Could you check a few things on this model? Use its own coordinates, in mm. A direction names the side the tool comes from. Round coordinates to 2 decimals unless told otherwise and drop trailing zeros. Loops run counter-clockwise (first coordinate to the right, second up) from the corner with the lowest first, then second, coordinate; pieces in that order, holes last. Notation, with made-up numbers: (32.25, 87) -> (83.25, 87) arc R29 cw to (83.25, 110) -> close; hole circle Ø8 at (-21, 80.5). An arc over 180 degrees is marked (long way). One line per item, written item: value.
from build123d import *
from build123d.topology import SkipClean

# Parameters (mm, degrees)
SKETCH3_R           = 122.5
SKETCH3_R_2         = 118.5
EXTRUDE_THIN1_DEPTH = 192
SKETCH3_3_R         = 122.5
BOSS_EXTRUDE4_DEPTH = 10
SKETCH11_R          = 5
BOSS_EXTRUDE5_DEPTH = 20
SKETCH13_R          = 27.5
CUT_EXTRUDE2_DEPTH  = 9
CIRPATTERN1_COUNT   = 6
SKETCH23_R          = 12.5
SKETCH23_R_2        = 10.5
EXTRUDE_THIN2_DEPTH = 9


with BuildPart() as part:
    # Sketch3 → Extrude-Thin1 (new body)
    with BuildSketch(Plane(origin=(0, 0, 0), x_dir=(1, 0, 0), z_dir=(0, 1, 0))):
        Circle(SKETCH3_R)
        Circle(SKETCH3_R_2, mode=Mode.SUBTRACT)
    extrude(amount=EXTRUDE_THIN1_DEPTH)

    # Sketch9 → Revolve2 (revolve)
    with BuildSketch(Plane.XY, mode=Mode.PRIVATE) as revolve2_sk:
        with BuildLine():
            Line((121.305664583, 189.351586859), (121.305664583, 192))
            Line((121.305664583, 192), (118.5, 192))
            ThreePointArc((118.5, 192), (122.710443221, 193.650108285), (121.305664583, 189.351586859))
        make_face()
    revolve(revolve2_sk.sketch.rotate(Axis((0, -1000, 0), (0, 1, 0)), 180), axis=Axis((0, -1000, 0), (0, 1, 0)))


with BuildPart() as body_2:
    # Sketch3_3 → Boss-Extrude4 (new body)
    with BuildSketch(Plane(origin=(0, 0, 0), x_dir=(1, 0, 0), z_dir=(0, 1, 0))):
        with Locations(Location((0, 0, 0), (0, 0, 270))):
            Circle(SKETCH3_3_R)
    extrude(amount=-BOSS_EXTRUDE4_DEPTH)


    with SkipClean():  # the faces are left unmerged after this step: merging them gives an invalid solid
        add(part.part)  # Boss-Extrude5 merges part
        # Sketch11 → Boss-Extrude5 (add)
        with BuildSketch(Plane(origin=(0, 0, 0), x_dir=(1, 0, 0), z_dir=(0, 1, 0))):
            with Locations(Location((0, 0, 0), (0, 0, 270))):
                Circle(SKETCH11_R)
        extrude(amount=BOSS_EXTRUDE5_DEPTH)

    # Sketch13 → Cut-Extrude2 (cut)
    with SkipClean():  # the faces are left unmerged after this step: merging them gives an invalid solid
        with BuildSketch(Plane.XZ.offset(10)):
            with Locations(Location((0, 0, 0), (0, 0, 270))):
                Circle(SKETCH13_R)
        extrude(amount=-CUT_EXTRUDE2_DEPTH, mode=Mode.SUBTRACT)

    # Sketch15 for Loft10 → Loft10 section 0
    with SkipClean():  # the faces are left unmerged after this step: merging them gives an invalid solid
        with BuildSketch(Plane.XZ.offset(1)):
            with BuildLine():
                Line((0, -15), (0, -27.124270964))
                # circular arc as an exact rational Bezier (weights 1, cos(half-angle), 1)
                Bezier((0, -27.124270964), (2.164566304, -27.124270964), (4.301737718, -26.780984447), weights=[1, 0.996830963, 1])
                Line((4.301737718, -26.780984447), (6.447780139, -13.543490366))
                Bezier((6.447780139, -13.543490366), (3.388397874, -15), (0, -15), weights=[1, 0.975422821, 1])
            make_face()
        # Sketch19 for Loft10 → Loft10 section 1
        with BuildSketch(Plane(origin=(0, -9, 0), x_dir=(1, 0, 0), z_dir=(0, 1, 0))):
            with BuildLine():
                Line((-0.43008531, 27.094099047), (-0.43008531, 14.993980537))
                Bezier((-0.43008531, 14.993980537), (0.03482173, 15.006996741), (0.49966504, 14.99187476), weights=[1, 0.999542352, 1])
                Line((0.49966504, 14.99187476), (0.49966504, 27.159324131))
                Line((0.49966504, 27.159324131), (-0.43008531, 27.094099047))
            make_face()
        loft10 = loft()

    # CirPattern1: Loft10 ×6 about axis
    with SkipClean():  # the faces are left unmerged after this step: merging them gives an invalid solid
        cirpattern1_axis = Axis((0, -1000, 0), (0, 1, 0))
        for i in range(1, CIRPATTERN1_COUNT):
            add(loft10.rotate(cirpattern1_axis, i * 360 / CIRPATTERN1_COUNT))

    # Sketch23 → Extrude-Thin2 (add)
    with SkipClean():  # the faces are left unmerged after this step: merging them gives an invalid solid
        with BuildSketch(Plane(origin=(0, -1, 0), x_dir=(-1, 0, 0), z_dir=(0, -1, 0))):
            Circle(SKETCH23_R)
            Circle(SKETCH23_R_2, mode=Mode.SUBTRACT)
        extrude(amount=EXTRUDE_THIN2_DEPTH)


solid = body_2.part
(1) For faces 3 (the face through (18.3, -9, -10.5)), 4 (the face through (0, 20, 0)), which set-ups out of +Z, -Z, +X, -X, +Y, -Y let a thin tool reach every point of the face, with its end or its side?
Recorded:
face 3: -Y
face 4: +Y
(2) If I drill on L1, parallel to X at y = -4, z = 0; L2, parallel to X at y = 109, z = 0; L3, parallel to Z at x = 47, y = 97, over which ranges is the centre line in solid material (lowest first)?
Recorded:
L1: -122.5 to -27.5, -12.5 to -10.5, 10.5 to 12.5, 27.5 to 122.5
L2: -122.5 to -118.5, 118.5 to 122.5
L3: -113.12 to -108.78, 108.78 to 113.12
(3) If we section it at A-A, the plane y = 35: Please give me the cut outline in (x, z), then the cut area to 3 significant figures.
Recorded:
outline: circle Ø245 at (0, 0); hole circle Ø237 at (0, 0)
area: 3,030 mm²
(4) Thinking about a two-plate mould opening in Z: for faces 1 (the face through (-10, -5.4, -3.2)), 2 (the face through (29, -10, -2)), which applies, released by +Z, released by -Z, zero draft, split by the parting line, or undercut?
Recorded:
face 1: undercut
face 2: zero draft
(5) I'm going to push flat-ended pins straight in: pin 1 Ø24 at (x, z) = (0, 0) entering from +Y; pin 2 Ø2 at (x, z) = (17, -10) entering from -Y; pin 3 Ø8 at (y, z) = (38, 12) entering from -X. Where does each tip first touch, or does it pass through?
Recorded:
pin 1: y = 20
pin 2: y = -9
pin 3: x = -122.24
